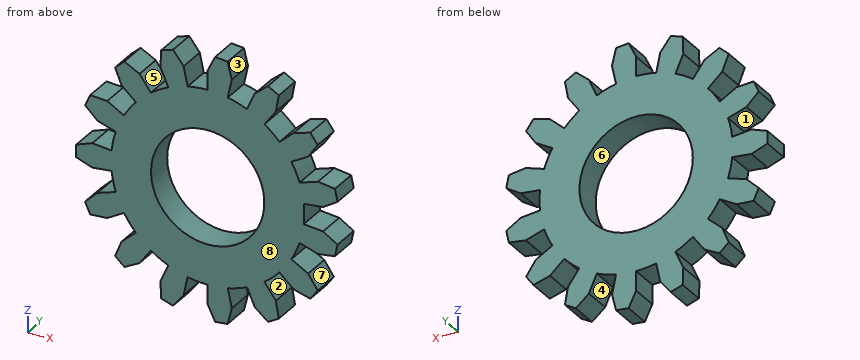
Autodesk Inventor part; units mm, degrees
ref_plane "YZ Plane" through (0, 0, 0) normal (1, 0, 0) x (0, 1, 0)
ref_plane "XZ Plane" through (0, 0, 0) normal (0, 1, 0) x (-1, 0, 0)
ref_plane "XY Plane" through (0, 0, 0) normal (0, 0, 1) x (1, 0, 0)
sketch "スケッチ1" plane through (0, 0, 0) normal (0, 1, 0) x (-1, 0, 0)
  circle A0 centre (0, 0) radius 22.5 construction
  circle A1 centre (0, 0) radius 25.5 construction
  line L0 (25.5, 1.2181) -> (25.5, -1.2181)
  line L1 (25.5, 1.2181) -> (22.3764, 2.355)
  line L2 (25.5, -1.2181) -> (22.3764, -2.355)
  line L3 (35.7, 0) -> (-35.7, 0)
  circle A2 centre (0, 0) radius 18.75
  line L4 (22.3764, -2.355) -> (18.647, -1.9625)
  line L5 (22.3764, 2.355) -> (18.647, 1.9625)
  line L6 (19.484, 11.2527) -> (16.2367, 9.3773)
  line L7 (22.8, 11.4846) -> (19.484, 11.2527)
  line L8 (22.8, 11.4846) -> (23.7909, 9.259)
  line L9 (23.7909, 9.259) -> (21.3997, 6.9499)
  line L10 (21.3997, 6.9499) -> (17.8331, 5.7916)
  line L11 (13.2226, 18.2047) -> (11.0189, 15.1706)
  line L12 (16.1576, 19.7653) -> (13.2226, 18.2047)
  line L13 (16.1576, 19.7653) -> (17.9681, 18.1351)
  line L14 (17.9681, 18.1351) -> (16.7229, 15.0531)
  line L15 (16.7229, 15.0531) -> (13.9357, 12.5443)
  line L16 (4.675, 22.009) -> (3.8958, 18.3408)
  line L17 (6.7214, 24.6284) -> (4.675, 22.009)
  line L18 (6.7214, 24.6284) -> (9.0384, 23.8755)
  line L19 (9.0384, 23.8755) -> (9.1544, 20.5535)
  line L20 (9.1544, 20.5535) -> (7.6287, 17.1279)
  line L21 (-4.6811, 22.0077) -> (-3.9009, 18.3397)
  line L22 (-3.8769, 25.233) -> (-4.6811, 22.0077)
  line L23 (-3.8769, 25.233) -> (-1.454, 25.4876)
  line L24 (-1.454, 25.4876) -> (0.0031, 22.5)
  line L25 (0.0031, 22.5) -> (0.0026, 18.75)
  line L26 (-13.2277, 18.201) -> (-11.0231, 15.1675)
  line L27 (-13.8049, 21.4746) -> (-13.2277, 18.201)
  line L28 (-13.8049, 21.4746) -> (-11.6951, 22.6927)
  line L29 (-11.6951, 22.6927) -> (-9.1487, 20.556)
  line L30 (-9.1487, 20.556) -> (-7.6239, 17.13)
  line L31 (-19.4871, 11.2473) -> (-16.2393, 9.3727)
  line L32 (-21.3459, 14.0031) -> (-19.4871, 11.2473)
  line L33 (-21.3459, 14.0031) -> (-19.9139, 15.974)
  line L34 (-19.9139, 15.974) -> (-16.7187, 15.0578)
  line L35 (-16.7187, 15.0578) -> (-13.9322, 12.5481)
  line L36 (-22.3771, 2.3488) -> (-18.6476, 1.9573)
  line L37 (-25.196, 4.1103) -> (-22.3771, 2.3488)
  line L38 (-25.196, 4.1103) -> (-24.6895, 6.4932)
  line L39 (-24.6895, 6.4932) -> (-21.3978, 6.9559)
  line L40 (-21.3978, 6.9559) -> (-17.8315, 5.7965)
  line L41 (-21.3978, -6.9559) -> (-17.8315, -5.7965)
  line L42 (-24.6895, -6.4932) -> (-21.3978, -6.9559)
  line L43 (-24.6895, -6.4932) -> (-25.196, -4.1103)
  line L44 (-25.196, -4.1103) -> (-22.3771, -2.3488)
  line L45 (-22.3771, -2.3488) -> (-18.6476, -1.9573)
  line L46 (-16.7187, -15.0578) -> (-13.9322, -12.5481)
  line L47 (-19.9139, -15.974) -> (-16.7187, -15.0578)
  line L48 (-19.9139, -15.974) -> (-21.3459, -14.0031)
  line L49 (-21.3459, -14.0031) -> (-19.4871, -11.2473)
  line L50 (-19.4871, -11.2473) -> (-16.2393, -9.3727)
  line L51 (-9.1487, -20.556) -> (-7.6239, -17.13)
  line L52 (-11.6951, -22.6927) -> (-9.1487, -20.556)
  line L53 (-11.6951, -22.6927) -> (-13.8049, -21.4746)
  line L54 (-13.8049, -21.4746) -> (-13.2277, -18.201)
  line L55 (-13.2277, -18.201) -> (-11.0231, -15.1675)
  line L56 (0.0031, -22.5) -> (0.0026, -18.75)
  line L57 (-1.454, -25.4876) -> (0.0031, -22.5)
  line L58 (-1.454, -25.4876) -> (-3.8769, -25.233)
  line L59 (-3.8769, -25.233) -> (-4.6811, -22.0077)
  line L60 (-4.6811, -22.0077) -> (-3.9009, -18.3397)
  line L61 (9.1544, -20.5535) -> (7.6287, -17.1279)
  line L62 (9.0384, -23.8755) -> (9.1544, -20.5535)
  line L63 (9.0384, -23.8755) -> (6.7214, -24.6284)
  line L64 (6.7214, -24.6284) -> (4.675, -22.009)
  line L65 (4.675, -22.009) -> (3.8958, -18.3408)
  line L66 (16.7229, -15.0531) -> (13.9357, -12.5443)
  line L67 (17.9681, -18.1351) -> (16.7229, -15.0531)
  line L68 (17.9681, -18.1351) -> (16.1576, -19.7653)
  line L69 (16.1576, -19.7653) -> (13.2226, -18.2047)
  line L70 (13.2226, -18.2047) -> (11.0189, -15.1706)
  line L71 (21.3997, -6.9499) -> (17.8331, -5.7916)
  line L72 (23.7909, -9.259) -> (21.3997, -6.9499)
  line L73 (23.7909, -9.259) -> (22.8, -11.4846)
  line L74 (22.8, -11.4846) -> (19.484, -11.2527)
  line L75 (19.484, -11.2527) -> (16.2367, -9.3773)
  circle A3 centre (0, 0) radius 11
  point P0 (25.5, 0)
  point P1 (23.2954, 10.3718)
  point P2 (17.0628, 18.9502)
  point P3 (7.8799, 24.2519)
  point P4 (-2.6655, 25.3603)
  point P5 (-12.75, 22.0836)
  point P6 (-20.6299, 14.9885)
  point P7 (-24.9428, 5.3017)
  point P8 (-24.9428, -5.3017)
  point P9 (-20.6299, -14.9885)
  point P10 (-12.75, -22.0836)
  point P11 (-2.6655, -25.3603)
  point P12 (7.8799, -24.2519)
  point P13 (17.0628, -18.9502)
  point P14 (23.2954, -10.3718)
  point P15 (17.8331, 5.7916)
  point P16 (16.2367, 9.3773)
  point P17 (13.9357, 12.5443)
  point P18 (11.0189, 15.1706)
  point P19 (7.6287, 17.1279)
  point P20 (3.8958, 18.3408)
  point P21 (0.0026, 18.75)
  point P22 (-3.9009, 18.3397)
  point P23 (-7.6239, 17.13)
  point P24 (-11.0231, 15.1675)
  point P25 (-13.9322, 12.5481)
  point P26 (-16.2393, 9.3727)
  point P27 (-17.8315, 5.7965)
  point P28 (-18.6476, 1.9573)
  point P29 (-18.6476, -1.9573)
  point P30 (-17.8315, -5.7965)
  point P31 (-16.2393, -9.3727)
  point P32 (-13.9322, -12.5481)
  point P33 (-11.0231, -15.1675)
  point P34 (-7.6239, -17.13)
  point P35 (-3.9009, -18.3397)
  point P36 (0.0026, -18.75)
  point P37 (3.8958, -18.3408)
  point P38 (7.6287, -17.1279)
  point P39 (11.0189, -15.1706)
  point P40 (13.9357, -12.5443)
  point P41 (16.2367, -9.3773)
  point P42 (17.8331, -5.7916)
  dimension "d5" = 37.5
  dimension "d0" = 45
  dimension "d1" = 51
  dimension "d3" = 20
  dimension "d4" = 20
  dimension "d14" = 4.71
  dimension "d18" = 360
  dimension "d23" = 22
extrude "押し出し1" add sketch "スケッチ1" along normal blind 5.5 contours L0 L3 A2 L5 L1 | L0 L2 L4 A2 L3 | A2 L3 A3 | L3 A3 A2 | A2 L6 L7 L8 L9 L10 | L71 L72 L73 L74 L75 A2 | A2 L11 L12 L13 L14 L15 | L36 L37 L38 L39 L40 A2 | A2 L41 L42 L43 L44 L45 | L66 L67 L68 L69 L70 A2 | A2 L16 L17 L18 L19 L20 | L31 L32 L33 L34 L35 A2 | A2 L46 L47 L48 L49 L50 | L61 L62 L63 L64 L65 A2 | A2 L21 L22 L23 L24 L25 | L26 L27 L28 L29 L30 A2 | A2 L51 L52 L53 L54 L55 | L56 L57 L58 L59 L60 A2
properties part number "M3_15"
The listing builds one solid part. Answer for the finished solid, in the listing's coordinates (mm). Face numbers are marked on the shaded views. A direction names the side the tool comes from. Round coordinates to 2 decimals unless told otherwise and drop trailing zeros. Write each loop counter-clockwise with the first axis right and the second up, starting at its lowest first coordinate (ties: lowest second). Pieces come first, ordered by that corner, then holes. Notation, with made-up numbers: M 9,-4.5 L 52,-4.5 A25 ccw 52,32.5 Z; hole C 56,-20 d3. An arc over 180 degrees is marked long. Write each question's results on one line, items separated by ' | '. Start each with the question number.
(1) Find the intervals of material crossed by line 1 (X direction, y = 1.85, z = 0); line 2 (X direction, y = 3.5, z = 21.5); line 3 (X direction, y = 4.1, z = 19), in increasing order.
(2) The part is cut by section B-B, the plane x = -15.5. Write down the section's boundary in (y, z), and give its area (3 significant figures).
(3) Determine the mould class of the marked faces 5, 6, 7 and 8 for opening direction Z: +Z half, -Z half, draft (parallel to the pull), parting line (faces both ways), or undercut.
(4) Each of these flat-tipped pins is pushed along its axis until it touches: P1, Ø2, axis at y = 1, z = 10, coming from the -X side; P2, Ø1.1, axis at y = 2, z = 20, coming from the -X side; P3, Ø3, axis at y = 1.5, z = -19.5, coming from the -X side. Where does it stop, or does it pass through?
(5) The part is cut by section A-A, the plane z = 0. Write down the section's boundary in (x, y), and give its area (3 significant figures).
(6) For the marked faces 1, 2, 3 and 4, determine the directions among +Z, -Z, +X, -X, +Y, -Y from which every point of the face is accessible in a straight line to the end or side of a thin tool.
Worked answers:
1) line 1: x = -25.5 to -11, 11 to 18.75 | line 2: x = -9.12 to -4.57, 0 to 4.57, 10.27 to 13.76 | line 3: x = -17.01 to -14.72, -8.46 to -4.04, 0 to 4.04, 8.46 to 13.37
2) outline: M 0,-19.42 L 5.5,-19.42 L 5.5,-13.95 L 0,-13.95 Z; M 0,-10.55 L 5.5,-10.55 L 5.5,10.55 L 0,10.55 Z; M 0,13.95 L 5.5,13.95 L 5.5,19.42 L 0,19.42 Z | area: 176 mm²
3) face 5: +Z half | face 6: undercut | face 7: undercut | face 8: draft
4) P1: stops at x = -23.79 | P2: stops at x = -16.51 | P3: stops at x = -17.97
5) outline: M -25.5,0 L -11,0 L -11,5.5 L -25.5,5.5 Z; M 11,0 L 18.75,0 L 18.75,5.5 L 11,5.5 Z | area: 122 mm²
6) face 1: -X, +Y, -Y | face 2: +Y, -Y | face 3: +Z, +Y, -Y | face 4: -Z, +Y, -Y
